Source: CAD feature listing. Evaluate the final solid. Frame: model axes, mm. Face numbers are marked on the shaded views. A direction names the side the tool comes from. Round coordinates to 2 decimals unless told otherwise and drop trailing zeros. Loops run counter-clockwise (first coordinate to the right, second up) from the corner with the lowest first, then second, coordinate; pieces in that order, holes last. Notation, with made-up numbers: (57.5, 25) -> (111.5, 25) arc R13 cw to (111.5, 42) -> close; hole circle Ø11 at (25.5, -5.5). An arc over 180 degrees is marked (long way). Put each result on its own line as item: value. Start each with the question number.
1. Cut plane C-C (z = 3.5). Return the cut outline in (x, y), then the cut area to 3 significant figures.
2. Cut plane B-B (y = -3.5). Return the cut outline in (x, z).
3. Draft query along X for the marked faces 1, 2, 3 and 4. Return one class per face: pulls with the +X half, pulls with the -X half, needs draft (parallel to the pull), parting line crosses it, or undercut.
4. Set-up query: the marked faces 5 and 6. Return all of +Z, -Z, +X, -X, +Y, -Y with unobstructed straight access to the full face (end or side cutting, diameter ignored); none if empty.
5. Cut plane A-A (x = 5). Return the cut outline in (y, z), then the cut area to 3 significant figures.
6. Cut plane D-D (x = -5). Return the cut outline in (y, z).
7. Contact query for flat-ended pins moving along their axis: pin 1 (12 mm diameter, centred on x = -11, z = 13, fed in from +Y); pin 2 (8 mm diameter, centred on x = 6.5, y = 19.5, fed in from -Z); pin 3 (9 mm diameter, centred on x = -7.5, y = 0.5, fed in from +Z). Output: stop coordinate, or through.
8. Material intervals for L1, parallel to Y at x = 5, z = 2.55; L2, parallel to Y at x = 8.75, z = 2; L3, parallel to X at y = -2, z = 3, sorted ascending.
```python
from build123d import *

# Parameters (mm, degrees)
SKETCH_1_W          = 30
SKETCH_1_H          = 62
SKETCH_1_W_2        = 20.4
SKETCH_1_H_2        = 40.2
EXTRUDE_1_DEPTH     = 4.5
SKETCH_3_R          = 2.25
SKETCH_3_R_2        = 2.20649786
CUT_EXTRUDE_1_DEPTH = 35.731109974
SKETCH_5_W          = 30
SKETCH_5_H          = 4.5
EXTRUDE_3_DEPTH     = 20
SKETCH_6_W          = 30
SKETCH_6_H          = 30
EXTRUDE_4_DEPTH     = 5
SKETCH_7_R          = 1.55
CUT_EXTRUDE_2_DEPTH = 94.241621608
SKETCH_8_W          = 1.6
SKETCH_8_H          = 5
CUT_EXTRUDE_3_DEPTH = 2.6


with BuildPart() as part:
    # 草图1 → 凸台-拉伸1 (new body)
    with BuildSketch(Plane.XY):
        Rectangle(SKETCH_1_W, SKETCH_1_H)
        Rectangle(SKETCH_1_W_2, SKETCH_1_H_2, mode=Mode.SUBTRACT)
    extrude(amount=EXTRUDE_1_DEPTH)

    # 草图3 → 切除-拉伸1 (cut, through all)
    with BuildSketch(Plane(origin=(0, 0, 0), x_dir=(-1, 0, 0), z_dir=(0, 0, -1))):
        with Locations((-5, -24.8)):
            Circle(SKETCH_3_R)
        with Locations((5, -24.8)):
            Circle(SKETCH_3_R)
        with Locations((-5, 24.8)):
            Circle(SKETCH_3_R)
        with Locations((5, 24.8)):
            Circle(SKETCH_3_R_2)
    extrude(amount=-CUT_EXTRUDE_1_DEPTH, mode=Mode.SUBTRACT)

    # 草图5 → 凸台-拉伸3 (add)
    with BuildSketch(Plane.XZ.offset(31)):
        with Locations((0, 2.25)):
            Rectangle(SKETCH_5_W, SKETCH_5_H)
    extrude(amount=EXTRUDE_3_DEPTH)

    # 草图6 → 凸台-拉伸4 (add)
    with BuildSketch(Plane.XZ.offset(51)):
        with Locations((0, 15)):
            Rectangle(SKETCH_6_W, SKETCH_6_H)
    extrude(amount=EXTRUDE_4_DEPTH)

    # 草图7 → 切除-拉伸2 (cut, through all)
    with BuildSketch(Plane.XZ.offset(56)):
        with Locations(Location((10, 22, 0), (0, 0, 270))):
            Circle(SKETCH_7_R)
        with Locations(Location((-10, 22, 0), (0, 0, 270))):
            Circle(SKETCH_7_R)
    extrude(amount=-CUT_EXTRUDE_2_DEPTH, mode=Mode.SUBTRACT)

    # 草图8 → 切除-拉伸3 (cut)
    with BuildSketch(Plane.XY.offset(4.5)):
        with Locations((0, -22.6)):
            Rectangle(SKETCH_8_W, SKETCH_8_H)
        with Locations((0, 22.6)):
            Rectangle(SKETCH_8_W, SKETCH_8_H)
    extrude(amount=-CUT_EXTRUDE_3_DEPTH, mode=Mode.SUBTRACT)


solid = part.part
```
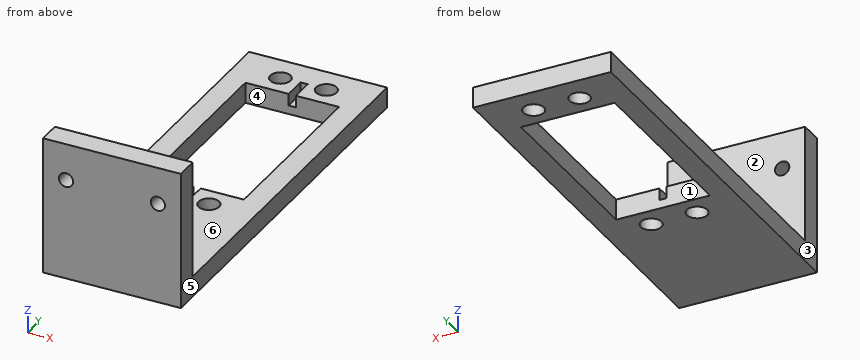
Solution:
1. outline: (-15, -56) -> (15, -56) -> (15, 31) -> (-15, 31) -> close; hole (-10.2, -20.1) -> (-0.8, -20.1) -> (-0.8, -25.1) -> (0.8, -25.1) -> (0.8, -20.1) -> (10.2, -20.1) -> (10.2, 20.1) -> (0.8, 20.1) -> (0.8, 25.1) -> (-0.8, 25.1) -> (-0.8, 20.1) -> (-10.2, 20.1) -> close; hole circle Ø4.5 at (-5, -24.8); hole circle Ø4.41 at (-5, 24.8); hole circle Ø4.5 at (5, -24.8); hole circle Ø4.5 at (5, 24.8)
1. area: 1,710 mm^2
2. outline: (-15, 0) -> (-10.2, 0) -> (-10.2, 4.5) -> (-15, 4.5) -> close; (10.2, 0) -> (15, 0) -> (15, 4.5) -> (10.2, 4.5) -> close
3. face 1: undercut
3. face 2: needs draft
3. face 3: pulls with the -X half
3. face 4: undercut
4. face 5: +Z, -Z, +X, +Y, -Y
4. face 6: +Z, +X, -X, +Y
5. outline: (-56, 0) -> (-27.05, 0) -> (-27.05, 4.5) -> (-51, 4.5) -> (-51, 30) -> (-56, 30) -> close; (-22.55, 0) -> (-20.1, 0) -> (-20.1, 4.5) -> (-22.55, 4.5) -> close; (20.1, 0) -> (22.55, 0) -> (22.55, 4.5) -> (20.1, 4.5) -> close; (27.05, 0) -> (31, 0) -> (31, 4.5) -> (27.05, 4.5) -> close
5. area: 298 mm^2
6. outline: (-56, 0) -> (-27.05, 0) -> (-27.05, 4.5) -> (-51, 4.5) -> (-51, 30) -> (-56, 30) -> close; (-22.55, 0) -> (-20.1, 0) -> (-20.1, 4.5) -> (-22.55, 4.5) -> close; (20.1, 0) -> (22.59, 0) -> (22.59, 4.5) -> (20.1, 4.5) -> close; (27.01, 0) -> (31, 0) -> (31, 4.5) -> (27.01, 4.5) -> close
7. pin 1: stops at y = -51
7. pin 2: stops at z = 0
7. pin 3: stops at z = 4.5
8. L1: y = -56 to -27.05, -22.55 to -20.1, 20.1 to 22.55, 27.05 to 31
8. L2: y = -56 to -20.1, 20.1 to 31
8. L3: x = -15 to -10.2, 10.2 to 15
